Input: part model. Units: mm. Frame: model coordinates. A direction names the side the tool comes from. Coordinates: 2 decimals unless noted, no trailing zeros. Write each loop counter-clockwise with the first axis right and the second up, starting at its lowest first coordinate (ties: lowest second). Pieces come first, ordered by that corner, then holes. Notation, with made-up numbers: (39.5, -34) - (61.5, -34) arc R20 ccw to (61.5, -17) - close; hole circle Ø1 at (23, 48). An arc over 180 degrees is marked (long way). Use a Markdown table: item, result. Add a question column.
Q1. Material intervals for probe 1 along Y at (x, z) = (53, 1.5); probe 2 along X at (y, z) = (53, 2.2); probe 3 along X at (y, z) = (-5.5, 2), sorted ascending. Write a range as from..to.
Q2. Section query A-A (x = 0). Return the cut outline in (y, z), then the cut area to 3 significant figures.
Q3. Section query C-C (z = 6.25). Return the cut outline in (x, y), then the cut area to 3 significant figures.
Q4. Set-up query: faces 1 (the face through (-27.34, -99.57, 3)), 2 (the face through (-104.3, 25.6, 1.5)). Return all of +Z, -Z, +X, -X, +Y, -Y with unobstructed straight access to the full face (end or side cutting, diameter ignored); none if empty.
Q5. Pin query (flat end, axial travel): P1, Ø1, axis at y = 43, z = 11, coming from the -X side; P2, Ø12, axis at x = -78.5, y = -36.5, coming from the +Z side; P3, Ø15, axis at x = 27.43, y = 102.39, coming from the +Z side; P4, Ø14.5, axis at x = -94.5, y = -52, coming from the +Z side. Return the tip coordinate at first contact, or that it passes through.
Q6. Mould query, pull axis Y, two halves, no side actions, for faces 3 (the face through (55.648, -91.913, 1.479)), 4 (the face through (-103.46, 42.9, 4.56)), 5 (the face through (-42, -92, 0)). Classes: released by +Y, released by -Y, zero draft, split by the parting line, or undercut.
from build123d import *

# Parameters (mm, degrees)
SKETCH3_R          = 2.65
CUT_EXTRUDE1_DEPTH = 160.100597108
CUT_EXTRUDE2_START = -3
SKETCH4_R          = 6.5
CUT_EXTRUDE2_DEPTH = 157.100597258
CIRPATTERN1_COUNT  = 8


with BuildPart() as part:
    # Sketch2 → Revolve1 (revolve)
    with BuildSketch(Plane(origin=(0, 0, 0), x_dir=(1, 0, 0), z_dir=(0, 1, 0))):
        with BuildLine():
            Line((-100, 0), (-112, 0))
            Line((-112, 0), (-112, -9))
            ThreePointArc((-112, -9), (-102.096675088, -13.469639994), (-91.339745962, -15))
            Line((-91.339745962, -15), (-100, 0))
        make_face()
    revolve(axis=Axis((0, 0, 0), (0, 0, 1)))

    # Sketch3 → Cut-Extrude1 (cut, through all)
    with BuildSketch(Plane(origin=(0, 0, 0), x_dir=(-1, 0, 0), z_dir=(0, 0, -1))):
        with Locations((-102.388137587, -27.434818781)):
            Circle(SKETCH3_R)
    cut_extrude1 = extrude(amount=-CUT_EXTRUDE1_DEPTH, mode=Mode.SUBTRACT)

    # Sketch4 → Cut-Extrude2 (cut, through all)
    with BuildSketch(Plane(origin=(0, 0, 0), x_dir=(-1, 0, 0), z_dir=(0, 0, -1)).offset(CUT_EXTRUDE2_START)):
        with Locations((-102.388137587, -27.434818781)):
            Circle(SKETCH4_R)
    cut_extrude2 = extrude(amount=-CUT_EXTRUDE2_DEPTH, mode=Mode.SUBTRACT)

    # CirPattern1: Cut-Extrude1, Cut-Extrude2 ×8 about axis
    cirpattern1_axis = Axis((0, 0, 0), (0, 0, 1))
    add([cut_extrude1.rotate(cirpattern1_axis, i * 360 / CIRPATTERN1_COUNT) for i in range(1, CIRPATTERN1_COUNT)], mode=Mode.SUBTRACT)
    add([cut_extrude2.rotate(cirpattern1_axis, i * 360 / CIRPATTERN1_COUNT) for i in range(1, CIRPATTERN1_COUNT)], mode=Mode.SUBTRACT)


solid = part.part
Values follow:
| question | item | result |
|---|---|---|
| 1 | probe 1 | -98.67..-94.45, -89.15..-83.78, 83.78..98.67 |
| 1 | probe 2 | -98.67..-83.3, 83.3..89.15, 94.45..98.67 |
| 1 | probe 3 | -111.86..-98.69, 98.69..111.86 |
| 2 | outline | (-112, 0) - (-100, 0) - (-91.34, 15) arc R38.57 ccw to (-112, 9) - close; (91.34, 15) - (100, 0) - (112, 0) - (112, 9) arc R38.57 ccw to start |
| 2 | area | 410 mm2 |
| 3 | outline | (-108.82, 26.5) arc R112 ccw to (-98.25, -53.76) arc R6.5 cw (long way) to (-95.68, -58.21) arc R112 ccw to (-31.46, -107.49) arc R6.5 cw (long way) to (-26.5, -108.82) arc R112 ccw to (53.76, -98.25) arc R6.5 cw (long way) to (58.21, -95.68) arc R112 ccw to (107.49, -31.46) arc R6.5 cw (long way) to (108.82, -26.5) arc R112 ccw to (98.25, 53.76) arc R6.5 cw (long way) to (95.68, 58.21) arc R112 ccw to (31.46, 107.49) arc R6.5 cw (long way) to (26.5, 108.82) arc R112 ccw to (-53.76, 98.25) arc R6.5 cw (long way) to (-58.21, 95.68) arc R112 ccw to (-107.49, 31.46) arc R6.5 cw (long way) to start; hole circle Ø192.78 at (0, 0) |
| 3 | area | 9,170 mm2 |
| 4 | face 1 | +Z |
| 4 | face 2 | +Z, -Z |
| 5 | P1 | x = -100.64 |
| 5 | P2 | z = 15 |
| 5 | P3 | z = 14.33 |
| 5 | P4 | z = 13.81 |
| 6 | face 3 | undercut |
| 6 | face 4 | split by the parting line |
| 6 | face 5 | zero draft |
